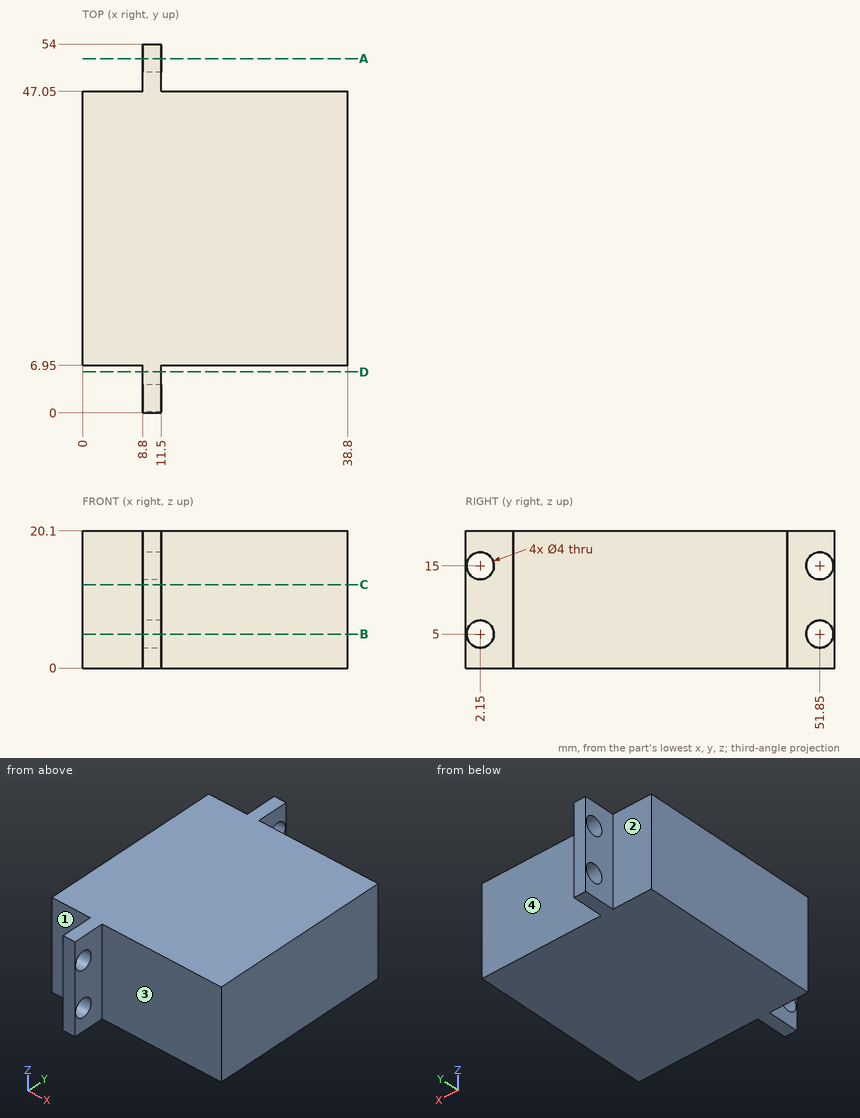
Answer from the drawing. Dimensions are ordinates in mm from the lowest x, y and z of the part. A direction names the side the tool comes from. Coordinates: 2 decimals unless noted, no trailing zeros. Write each loop counter-clockwise with the first axis right and the second up, starting at its lowest first coordinate (ties: lowest second). Pieces come first, ordered by that corner, then holes. Notation, with made-up numbers: M 49.25,-22 L 78.25,-22 A12 cw 78.25,-15 Z; hole C 68,70 d11. An arc over 180 degrees is marked long. Write item = value, one per line.
1. Straight lines are drawn through the part: line 1 (Y direction, x = 10.9, z = 5); line 2 (Z direction, x = 9, y = 2); line 3 (Z direction, x = 10, y = 51). For each, find the intervals that lie inside material, in ascending order. Write a range as from..to.
Solution:
line_1 = 0..0.15, 4.15..49.85, 53.85..54
line_2 = 0..3.01, 6.99..13.01, 16.99..20.1
line_3 = 0..3.19, 6.81..13.19, 16.81..20.1
2. The part is cut by section A-A (y = 51.85). Determine the outline of the cut face in (x, z).
Solution:
outline = M 8.8,0 L 11.5,0 L 11.5,3 L 8.8,3 Z; M 8.8,7 L 11.5,7 L 11.5,13 L 8.8,13 Z; M 8.8,17 L 11.5,17 L 11.5,20.1 L 8.8,20.1 Z
3. The part is cut by section C-C (z = 12.25). Determine the outline of the cut face in (x, y).
Solution:
outline = M 0,6.95 L 8.8,6.95 L 8.8,0 L 11.5,0 L 11.5,6.95 L 38.8,6.95 L 38.8,47.05 L 11.5,47.05 L 11.5,54 L 8.8,54 L 8.8,47.05 L 0,47.05 Z
4. The part is cut by section B-B (z = 5). Determine the outline of the cut face in (x, y), then the cut area to 3 significant figures.
Solution:
outline = M 0,6.95 L 8.8,6.95 L 8.8,4.15 L 11.5,4.15 L 11.5,6.95 L 38.8,6.95 L 38.8,47.05 L 11.5,47.05 L 11.5,49.85 L 8.8,49.85 L 8.8,47.05 L 0,47.05 Z; M 8.8,0 L 11.5,0 L 11.5,0.15 L 8.8,0.15 Z; M 8.8,53.85 L 11.5,53.85 L 11.5,54 L 8.8,54 Z
area = 1,570 mm2
5. Flat-ended cylindrical pins translate along their axes: pin 1 (3.5 mm diameter, centred on y = 2, z = 12, fed in from -X); pin 2 (3.5 mm diameter, centred on y = 2.15, z = 15, fed in from +X); pin 3 (2 mm diameter, centred on y = 51.5, z = 8, fed in from +X); pin 4 (2.5 mm diameter, centred on x = 5, z = 7.5, fed in from -Y). Find the tip coordinate at first contact, or state that the pin passes through.
Solution:
pin_1 = 8.8
pin_2 = through
pin_3 = 11.5
pin_4 = 6.95
6. The part is cut by section D-D (y = 6). Determine the outline of the cut face in (x, z).
Solution:
outline = M 8.8,0 L 11.5,0 L 11.5,20.1 L 8.8,20.1 Z
7. For the marked faces 1, 2, 3 and 4, determine the directions among +Z, -Z, +X, -X, +Y, -Y from which every point of the face is accessible in a straight line to the end or side of a thin tool.
Solution:
face_1 = +Z, -Z, -X, -Y
face_2 = +Z, -Z, -X, +Y
face_3 = +Z, -Z, +X, -Y
face_4 = +Z, -Z, +X, +Y
